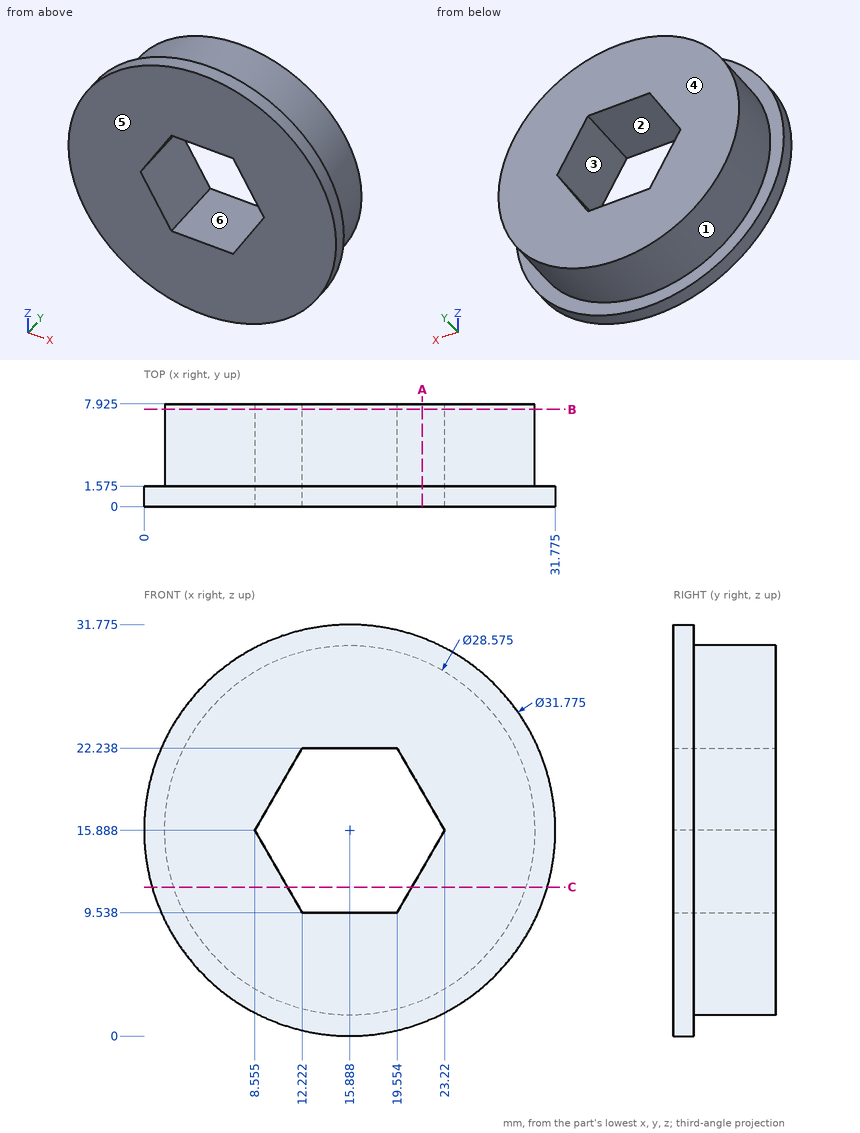
For this review, use the dimensioned drawing (mm, ordinates from the lowest corner) and the shaded views. A direction names the side the tool comes from. Give positions to 0.01 mm unless a question says otherwise; leave off trailing zeros. Order: outer loops, then holes, each group sorted by start corner. A loop starts at its lowest first (then second) coordinate and runs counter-clockwise, first axis right, second up.
1) For the marked faces 5 and 6, list the 3-axis set-ups (+Z, -Z, +X, -X, +Y, -Y) from which the entire face can be reached by the end or side of a thin tool; tool diameter is ignored.
2) Take a section at C-C (z = 11.5). Give the boundary of the cut face in (x, y) (1 decimal), then the cut area to 3 significant figures.
3) Wall thickness on line 1 (Y direction, x = 20.5, z = 2) (1 decimal); line 2 (Z direction, x = 23, y = 4.5) (1 decimal); line 3 (Z direction, x = 14, y = 0.5): over which ranges is each line inside the solid? List them lowest first.
4) Take a section at A-A (x = 21.5). Give the boundary of the cut face in (y, z) (1 decimal).
5) Insertion check: pin 1 (2 mm diameter, centred on x = 15.5, y = 3.5, fed in from +Z) (1 decimal); pin 2 (6 mm diameter, centred on x = 13, z = 17, fed in from -Y); pin 3 (3 mm diameter, centred on y = 1, z = 10, fed in from +X); pin 4 (2 mm diameter, centred on x = 14, y = 3, fed in from -Z). Each pin has a flat end and moves straight along its axis. Give the tip position at first contact, or say it passes through.
6) The part is to be moulded in two halves that separate along Z. For the marked faces 1, 2, 3 and 4, say which applies: released by +Z, released by -Z, zero draft, split by the parting line, or undercut.
7) Take a section at B-B (y = 7.5). Give the boundary of the cut face in (x, z) (1 decimal).
Derived:
1. face 5: +Z, -Z, +X, -X, -Y
1. face 6: +Y, -Y
2. outline: (0.6, 0) - (11.1, 0) - (11.1, 7.9) - (2.3, 7.9) - (2.3, 1.6) - (0.6, 1.6) - close; (20.7, 0) - (31.2, 0) - (31.2, 1.6) - (29.5, 1.6) - (29.5, 7.9) - (20.7, 7.9) - close
2. area: 145 mm2
3. line 1: y = 0 to 1.6
3. line 2: z = 3.5 to 15.5, 16.3 to 28.3
3. line 3: z = 0.11 to 9.54, 22.24 to 31.66
4. outline: (0, 1) - (1.6, 1) - (1.6, 2.7) - (7.9, 2.7) - (7.9, 12.9) - (0, 12.9) - close; (0, 18.9) - (7.9, 18.9) - (7.9, 29) - (1.6, 29) - (1.6, 30.8) - (0, 30.8) - close
5. pin 1: stops at z = 30.2
5. pin 2: passes through
5. pin 3: stops at x = 31.16
5. pin 4: stops at z = 1.63
6. face 1: split by the parting line
6. face 2: undercut
6. face 3: undercut
6. face 4: zero draft
7. outline: circle Ø28.6 at (15.9, 15.9); hole (8.6, 15.9) - (12.2, 9.5) - (19.6, 9.5) - (23.2, 15.9) - (19.6, 22.2) - (12.2, 22.2) - close
